from build123d import *

# Parameters (mm, degrees)
F1_DEPTH = 63.5
F2_DEPTH = 25.4
F3_DEPTH = 15.875
F0_W     = 25.4
F0_H     = 19.05
F4_DEPTH = 25.4
F6_R     = 6.35


with BuildPart() as f1:
    # F0 (on Front) → F1 (new body, symmetric)
    with BuildSketch(Plane.XZ):
        Polygon((22.225, 9.525), (-41.275, 9.525), (-41.275, -9.525), (41.275, -9.525), (41.275, 9.525), align=None)
    extrude(amount=F1_DEPTH, both=True)

    # F0 (on Front) → F2 (join, symmetric)
    with BuildSketch(Plane.XZ):
        with BuildLine():
            Line((22.225, 27.0002), (22.225, 9.525))
            Line((22.225, 9.525), (41.275, 9.525))
            Line((41.275, 9.525), (41.275, 27.0002))
            ThreePointArc((41.275, 27.0002), (45.9246798487, 38.2255201513), (57.15, 42.8752))
            Line((57.15, 42.8752), (60.325, 42.8752))
            Line((60.325, 42.8752), (60.325, 61.9252))
            Line((60.325, 61.9252), (57.15, 61.9252))
            add(Edge.make_bspline(
                [(56.7658276627, 61.9230870029), (56.8938039219, 61.92387202), (57.0218614604, 61.9245763394), (57.15, 61.9252)],
                knots=[111.2545269173, 111.2545269173, 111.2545269173, 111.2545269173, 111.5045361635, 111.5045361635, 111.5045361635, 111.5045361635], degree=3))
            ThreePointArc((56.7658276627, 61.9230870029), (32.3188417117, 51.5597033146), (22.225, 27.0002))
        make_face()
    extrude(amount=F2_DEPTH, both=True)

    # F0 (on Front) → F3 (join)
    with BuildSketch(Plane.XZ):
        with BuildLine():
            add(Edge.make_bspline(
                [(-41.275, 9.525), (-41.0380026786, 45.2441586696), (-0.1838187392, 61.5737531077), (56.7658276627, 61.9230870029)],
                knots=[0, 0, 0, 0, 111.2545269173, 111.2545269173, 111.2545269173, 111.2545269173], degree=3))
            Line((-41.275, 9.525), (22.225, 9.525))
            Line((22.225, 9.525), (22.225, 27.0002))
            ThreePointArc((22.225, 27.0002), (32.3188417117, 51.5597033146), (56.7658276627, 61.9230870029))
        make_face()
    extrude(amount=F3_DEPTH)

    # F0 (on Front) → F4 (join, symmetric)
    with BuildSketch(Plane.XZ):
        with Locations((73.025, 52.4002)):
            Rectangle(F0_W, F0_H)
    extrude(amount=F4_DEPTH, both=True)

    # F0 (on Front) → F5 (revolve)
    with BuildSketch(Plane.XZ):
        Polygon((85.725, 66.675), (85.725, 61.9252), (85.725, 42.8752), (85.725, 38.1), (111.125, 38.1), (111.125, 66.675), align=None)
    revolve(axis=Axis((85.725, 0, 52.3875), (0, 0, 1)))

    # F6
    f6_edges = [f1.edges().sort_by_distance(p)[0] for p in [
        (41.275, -63.5, 0),
        (-41.275, -63.5, 0),
        (41.275, 63.5, 0),
        (-41.275, 63.5, 0),
    ]]
    fillet(f6_edges, radius=F6_R)


solid = f1.part
Read the model definition and answer for the solid it produces. Units are mm, in the model's axes. A direction names the side the tool comes from. Give positions to 0.01 mm unless a question says otherwise; leave off trailing zeros. Loops run counter-clockwise (first coordinate to the right, second up) from the corner with the lowest first, then second, coordinate; pieces in that order, holes last. Notation, with made-up numbers: M -40,36.25 L -25,36.25 A17 cw -25,49.25 Z; hole C 82.5,76 d9. An arc over 180 degrees is marked long. Write each question's results on one line, items separated by ' | '.
1. Section C-C on y = -54 is taken. Give the vertices of the cut face in (x, z) (3 decimals).
Values:
outline: M -41.275,-9.525 L 41.275,-9.525 L 41.275,9.525 L -41.275,9.525 Z
2. The mould has two halves that part along X. Classify faces 1 (the face through (39.464, 61.59, 0.133)), 2 (the face through (1, -40, 9.525)), 3 (the face through (45.8, -0.4, 38.1)): pulls with the +X half, pulls with the -X half, needs draft (parallel to the pull), parting line crosses it, or undercut.
Values:
face 1: pulls with the +X half | face 2: needs draft | face 3: undercut
3. Section A-A on z = 4 is taken. Give the vertices of the cut face in (x, y) (3 decimals), plus the area to 3 significant figures.
Values:
outline: M -41.275,-57.15 A6.35 ccw -34.925,-63.5 L 34.925,-63.5 A6.35 ccw 41.275,-57.15 L 41.275,57.15 A6.35 ccw 34.925,63.5 L -34.925,63.5 A6.35 ccw -41.275,57.15 Z | area: 10,400 mm^2
4. Straight lines are drawn through the part: line 1 (Z direction, x = 21.5, y = -22) (3 decimals); line 2 (Z direction, x = 78.5, y = -6.5) (3 decimals); line 3 (Y direction, x = -15, z = 39.5) (3 decimals). For each, find the intervals that lie inside material, in ascending order. Write a range as [from, to].
Values:
line 1: z = [-9.525, 9.525] | line 2: z = [38.1, 66.675] | line 3: y = [-15.875, 0]
5. Given pin 1 (10 mm diameter, centred on y = -17.5, z = 39, fed in from +X); pin 2 (10 mm diameter, centred on x = 28.5, z = 27, fed in from +Y); pin 3 (11 mm diameter, centred on y = 14, z = 15.5, fed in from +X) (3 decimals), each flat-ended and moving along its own axis, determine where each tip first touches the part or whether it passes through.
Values:
pin 1: stops at x = 107.84 | pin 2: stops at y = 25.4 | pin 3: stops at x = 41.275
6. Section D-D on x = 92.5 is taken. Give the vertices of the cut face in (y, z) (3 decimals), plus the area to 3 significant figures.
Values:
outline: M -24.48,38.1 L 24.48,38.1 L 24.48,66.675 L -24.48,66.675 Z | area: 1,400 mm^2
7. Section B-B on x = 67 is taken. Give the vertices of the cut face in (y, z) (3 decimals), plus the area to 3 significant figures.
Values:
outline: M -25.4,42.875 L -17.162,42.875 L -17.162,38.1 L 17.162,38.1 L 17.162,42.875 L 25.4,42.875 L 25.4,61.925 L 17.162,61.925 L 17.162,66.675 L -17.162,66.675 L -17.162,61.925 L -25.4,61.925 Z | area: 1,290 mm^2
8. A tool of negligible diameter and unlimited length cuts with its end or side. For faces 4 (the face through (46, -25.4, 42)), 5 (the face through (-2, 0, 30)), 6 (the face through (60, 2, 42.875)), 7 (the face through (46, 25.4, 42)), 8 (the face through (32.59, -20.7, 51.83)), from which of +Z, -Z, +X, -X, +Y, -Y can it reach the whole face along a straight path? Write none if from no direction.
Values:
face 4: +Z, +X, -X, -Y | face 5: +Z, -X, +Y | face 6: -Z | face 7: +Z, +X, -X, +Y | face 8: +Z, -X, -Y
